Source: CAD feature listing. Evaluate the final solid. Frame: model axes, mm. Give positions to 0.01 mm unless a question says otherwise; leave off trailing zeros. Order: outer loops, then holes, each group sorted by start corner. A loop starts at its lowest first (then second) coordinate and runs counter-clockwise, first axis right, second up. Notation, with made-up numbers: M 15,14.25 L 68,14.25 A19 cw 68,29.25 Z; hole C 8.5,85 d3. An arc over 180 degrees is marked long. Use CSV: the item, a comma, the result in double quotes. Start each with the question number.
1. Section query B-B, the plane y = -106. Return the cut outline in (x, z).
2. Line query: line 1 along Y through (x, z) = (40.64, -0.35); line 2 along Y through (x, z) = (95, -0.6); line 3 along X through (y, z) = (29.5, 0.4). Output: solid intervals per line, ascending. Write a range as [from, to].
3. Pin query (flat end, axial travel): P1, Ø1.6, axis at y = -113.5, z = -0.5, coming from the -X side; P2, Ø1, axis at x = 59, z = 0, coming from the +Y side. Return the tip coordinate at first contact, or that it passes through.
4. Section query C-C, the plane x = 177. Return the cut outline in (y, z).
5. Section query A-A, the plane z = 0.35. Return the cut outline in (x, y).
from build123d import *

# Parameters (mm, degrees)
BOSS_EXTRUDE1_DEPTH      = 1.5875
BOSS_EXTRUDE1_DEPTH_BACK = 1.5875
SKETCH2_R                = 1.26619
CUT_EXTRUDE1_DEPTH       = 4.175


with BuildPart() as part:
    # Sketch1 → Boss-Extrude1 (new body, two sides)
    with BuildSketch(Plane.XY) as boss_extrude1_sk:
        Polygon((95.25, 127), (247.65, 76.2), (247.65, -76.2), (95.25, -127), (95.25, -76.2), (31.75, -76.2), (31.75, -38.1), (95.25, -38.1), (95.25, 38.1), (31.75, 38.1), (31.75, 76.2), (95.25, 76.2), align=None)
    extrude(amount=BOSS_EXTRUDE1_DEPTH)
    extrude(boss_extrude1_sk.sketch, amount=-BOSS_EXTRUDE1_DEPTH_BACK)

    # Sketch2 → Cut-Extrude1 (cut, through all)
    with BuildSketch(Plane.XY.offset(1.5875)):
        with Locations((40.64, 58.512580329)):
            Circle(SKETCH2_R)
        with Locations((40.64, -58.512580329)):
            Circle(SKETCH2_R)
    extrude(amount=-CUT_EXTRUDE1_DEPTH, mode=Mode.SUBTRACT)


solid = part.part
Result set:
1,outline,"M 95.25,-1.59 L 158.25,-1.59 L 158.25,1.59 L 95.25,1.59 Z"
2,line 1,"[-76.2, -59.78], [-57.25, -38.1], [38.1, 57.25], [59.78, 76.2]"
2,line 2,"[-76.2, -38.1], [38.1, 76.2]"
2,line 3,"[95.25, 247.65]"
3,P1,"x = 95.25"
3,P2,"y = 76.2"
4,outline,"M -99.75,-1.59 L 99.75,-1.59 L 99.75,1.59 L -99.75,1.59 Z"
5,outline,"M 31.75,-76.2 L 95.25,-76.2 L 95.25,-127 L 247.65,-76.2 L 247.65,76.2 L 95.25,127 L 95.25,76.2 L 31.75,76.2 L 31.75,38.1 L 95.25,38.1 L 95.25,-38.1 L 31.75,-38.1 Z; hole C 40.64,-58.51 d2.53; hole C 40.64,58.51 d2.53"
